Can you work these out from the model? Positions are in its coordinate system, mm. Face numbers are marked on the shaded views. A direction names the side the tool comes from. Coordinates: 2 decimals unless noted, no trailing zeros. Write each loop counter-clockwise with the first axis right and the second up, starting at its lowest first coordinate (ties: lowest second). Pieces come first, ordered by that corner, then holes.
```python
from build123d import *

# Parameters (mm, degrees)
F1_DEPTH  = 15
F3_DEPTH  = 15
F4_SIZE   = 2.5
F5_R      = 5.25
F6_DEPTH  = 15
F7_R      = 3
F8_DEPTH  = 35
F9_R      = 6.25
F10_DEPTH = 2


with BuildPart() as f1:
    # F0 (on Top) → F1 (new body)
    with BuildSketch(Plane.XY):
        Polygon((0, 62), (0, 0), (9, 0), (15, 30.5), (15, 48), (9.5, 48), (9.5, 62), align=None)
    extrude(amount=F1_DEPTH)

    # F2 (on face) → F3 (join)
    with BuildSketch(Plane(origin=(0, 0, 0), x_dir=(1, 0, 0), z_dir=(0, 0, -1))):
        Polygon((4.496674, -60), (9.5, -60), (9.5, -48), (15, -48), (15, -30.5), (9, 0), (0, 0), (0, -34), (4.496674, -34), align=None)
    extrude(amount=F3_DEPTH)

    # F4
    f4_edges = [f1.edges().sort_by_distance(p)[0] for p in [
        (4.496674, 60, -7.5),
    ]]
    chamfer(f4_edges, length=F4_SIZE)

    # F5 (on face) → F6 (cut)
    with BuildSketch(Plane(origin=(0, 0, 0), x_dir=(0, -1, 0), z_dir=(-1, 0, 0))):
        with Locations((-55.745944, 8.24335)):
            Circle(F5_R)
    extrude(amount=-F6_DEPTH, mode=Mode.SUBTRACT)

    # F7 (on face) → F8 (cut)
    with BuildSketch(Plane.XY.offset(15)):
        with Locations((7, 30)):
            Circle(F7_R)
    extrude(amount=-F8_DEPTH, mode=Mode.SUBTRACT)

    # F9 (on face) → F10 (cut)
    with BuildSketch(Plane(origin=(0, 0, -15), x_dir=(1, 0, 0), z_dir=(0, 0, -1))):
        with Locations((7, -30)):
            Circle(F9_R)
    extrude(amount=-F10_DEPTH, mode=Mode.SUBTRACT)


solid = f1.part
```
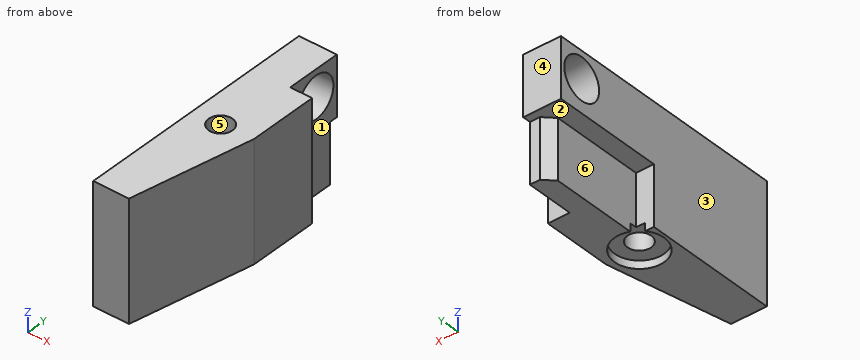
1. If I drill on L1, parallel to Y at x = 7, z = -2.5; L2, parallel to Y at x = 5, z = 11.5; L3, parallel to Y at x = 7, z = 0.75, over which ranges is the centre line in solid material (lowest first)?
2. If we section it at C-C, the plane z = 4.75: List the corners of the cut face in (x, y) for me (3 decimals), plus the area to 3 significant figures.
3. If we section it at D-D, the plane z = 11.5: List the corners of the cut face in (x, y) for me.
4. If we section it at A-A, the plane x = 5.25: List the corners of the cut face in (y, z) for me, plus the area to 3 significant figures.
5. If we section it at B-B, the plane z = -10: List the corners of the cut face in (x, y) for me, plus the area to 3 significant figures.
6. We'd pull the mould along Y, two halves only. Please class the marked faces 4, 5 and 6: released by +Y, released by -Y, zero draft, split by the parting line, or undercut.
7. I'm going to push flat-ended pins straight in: P1, Ø0.8, axis at x = 9, z = -8.5, coming from the +Y side; P2, Ø6.5, axis at y = 55.75, z = 8.24, coming from the -X side; P3, Ø12, axis at y = 43, z = -9.5, coming from the -X side; P4, Ø2, axis at x = 2.5, z = -8.5, coming from the +Y side. Where does each tip first touch, or does it pass through?
8. Which directions (+Z, -Z, +X, -X, +Y, -Y) give clear straight access to the entire face, cutting with the end or side of a thin tool? Please do the marked faces 1, 2 and 3.
Answers:
1. L1: y = 0 to 27, 33 to 60
1. L2: y = 0 to 27.76, 32.24 to 51.63, 59.86 to 62
1. L3: y = 0 to 27, 33 to 62
2. outline: (0, 0) - (9, 0) - (15, 30.5) - (15, 48) - (9.5, 48) - (9.5, 51.827) - (0, 51.827) - close; (0, 59.665) - (9.5, 59.665) - (9.5, 62) - (0, 62) - close; hole circle Ø6 at (7, 30)
2. area: 659 mm2
3. outline: (0, 0) - (9, 0) - (15, 30.5) - (15, 48) - (9.5, 48) - (9.5, 51.63) - (0, 51.63) - close; (0, 59.86) - (9.5, 59.86) - (9.5, 62) - (0, 62) - close; hole circle Ø6 at (7, 30)
4. outline: (0, -15) - (24, -15) - (24, -13) - (27.56, -13) - (27.56, 15) - (0, 15) - close; (32.44, -13) - (36, -13) - (36, -15) - (58.25, -15) - (58.25, 0) - (62, 0) - (62, 15) - (32.44, 15) - close; hole circle Ø10.5 at (55.75, 8.24)
4. area: 1,560 mm2
5. outline: (0, 0) - (9, 0) - (15, 30.5) - (15, 48) - (9.5, 48) - (9.5, 60) - (7, 60) - (4.5, 57.5) - (4.5, 34) - (0, 34) - close; hole circle Ø6 at (7, 30)
5. area: 594 mm2
6. face 4: released by +Y
6. face 5: undercut
6. face 6: zero draft
7. P1: stops at y = 60
7. P2: passes through
7. P3: stops at x = 4.5
7. P4: stops at y = 34
8. face 1: +Z, -Z, +X, +Y
8. face 2: -Z, -X, +Y
8. face 3: +Z, -Z, -X, +Y, -Y
